Verification items for the finished model (mm, model axes). Give positions to 0.01 mm unless a question says otherwise; leave off trailing zeros. Loops run counter-clockwise (first coordinate to the right, second up) from the corner with the lowest first, then second, coordinate; pieces in that order, holes last. Notation, with made-up numbers: M -36,-10 L -7,-10 A29 ccw -7,17 Z; hole C 49,10.25 d2. An arc over 180 degrees is marked long. Use CSV: the item, a comma, the result in double quotes.
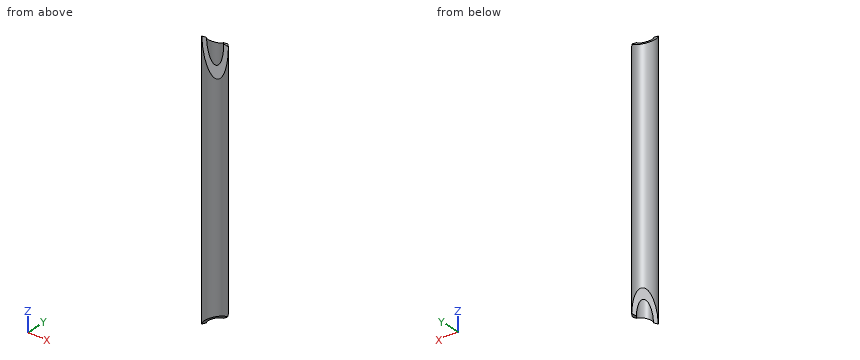
Autodesk Inventor part; units mm, degrees
ref_plane "Start Plane" through (0, 0, -3.37) normal (0, 0, 1) x (1, 0, 0)
ref_plane "End Plane" through (0, 0, 266.7183) normal (0, 0, 1) x (1, 0, 0)
ref_plane "Work Plane4" through (-6.8383, -8.1881, -6.8069) normal (0.3448, 0.4129, -0.843) x (0.2427, -0.9068, -0.3448)
ref_plane "Start Plane" through (0, 0, -3.37) normal (0, 0, 1) x (1, 0, 0)
ref_plane "End Plane" through (0, 0, 266.7183) normal (0, 0, 1) x (1, 0, 0)
sketch "Sketch" plane through (0, 0, 0) normal (0, 0, 1) x (1, 0, 0)
  circle A0 centre (0, 0) radius 6.9342
  circle A1 centre (0, 0) radius 10.668
  dimension "d0" = 21.336
  dimension "d1" = 3.7338
extrude "Body" add sketch "Sketch" along normal up to surface (270.0883 mm away) from surface at -3.37
sketch "Sketch3" plane through (0, 0, 0) normal (0, 0, 1) x (1, 0, 0)
  line L0 (0, 0) -> (10, 0)
ref_plane "Work Plane3" through (0, 0, 0) normal (0, -1, 0) x (1, 0, 0)
sketch "Sketch4" plane through (0, 0, 0) normal (0, -1, 0) x (1, 0, 0)
  line L0 (-2, -3.37) -> (12, -3.37)
  line L1 (-2, 266.7183) -> (12, 266.7183)
  dimension "d7" = 270.0883
ref_plane "Work Plane4" through (-6.8383, -8.1881, -6.8069) normal (0.3448, 0.4129, -0.843) x (0.2427, -0.9068, -0.3448)
split "Split1" plane through (-6.8383, -8.1881, -6.8069) removes the side toward (0.3448, 0.4129, -0.843)
ref_plane "Work Plane5" through (4.7044, -9.5747, -24.7602) normal (-0.405, 0.8243, -0.3957) x (0.7286, 0.5524, 0.405)
split "Split2" plane through (4.7044, -9.5747, -24.7602) removes the side toward (-0.405, 0.8243, -0.3957)
ref_plane "Work Plane6" through (-8.4798, 6.473, -10.5353) normal (0.5585, -0.4264, -0.7115) x (-0.0814, 0.8255, -0.5585)
split "Split3" plane through (-8.4798, 6.473, -10.5353) removes the side toward (0.5585, -0.4264, -0.7115)
ref_plane "Work Plane7" through (3.7346, -9.993, 272.7308) normal (-0.242, 0.6474, 0.7227) x (0.966, 0.0909, 0.242)
split "Split4" plane through (3.7346, -9.993, 272.7308) removes the side toward (-0.242, 0.6474, 0.7227)
ref_plane "Work Plane8" through (-8.4798, 6.473, 292.9957) normal (0.7502, -0.5727, 0.3305) x (0.577, 0.3229, -0.7502)
split "Split5" plane through (-8.4798, 6.473, 292.9957) removes the side toward (0.7502, -0.5727, 0.3305)
ref_plane "Work Plane9" through (-10.6242, -0.9653, 270.4444) normal (0.5935, 0.0539, 0.8031) x (0.8047, -0.0177, -0.5935)
split "Split6" plane through (-10.6242, -0.9653, 270.4444) removes the side toward (0.5935, 0.0539, 0.8031)
equation "\"d0\" = G_H"
equation "\"d1\" = G_T"
equation "\"d2\" = G_L"
equation "\"G_H\" = 21.336"
equation "\"G_T\" = 3.7338"
equation "\"G_L\" = 270.08826"
equation "\"G_OFFSET_START\" = 3.36995"
equation "\"G_OFFSET_END\" = 4.18997"
equation "\"d4\" = -G_OFFSET_START"
equation "\"d5\" = G_OFFSET_END + B_L"
equation "\"B_L\" = 262.52833"
properties part number "ANSI - 1/2 x 0.147 - 10.633" material "Steel, Mild"
(1) Scan lines: L1, parallel to X at y = 0, z = 73; L2, parallel to Y at x = -2, z = 64.5. Record each from-to range of solid material in increasing order. Write a range as from..to.
Calculated:
L1,"x = -10.67..-6.93, 6.93..10.67"
L2,"y = -10.48..-6.64, 6.64..10.48"
(2) Section check A-A on x = -2.5. Record the cut outline in (y, z).
Calculated:
outline,"M -10.37,4.25 L -6.47,1.91 L -6.47,257 L -10.37,250.23 Z; M 6.47,16.03 L 10.37,24.16 L 10.37,252.4 L 6.47,255.9 Z"
(3) Section check B-B on y = 0. Record the cut outline in (x, z), plus the area to 3 significant figures.
Calculated:
outline,"M -10.67,10.92 L -6.93,7.1 L -6.93,260.21 L -10.67,258.96 Z; M 6.93,5.44 L 10.67,8.37 L 10.67,238.32 L 6.93,246.79 Z"
area,"1,820 mm²"
(4) Depth check by flat-ended pin: pin 1 Ø3 at (x, z) = (-1.5, 31) entering from -Y; pin 2 Ø12 at (y, z) = (6.5, 175.5) entering from +X; pin 3 Ø3 at (y, z) = (7.5, 237.5) entering from +X; pin 4 Ø3 at (x, z) = (6.5, 217.5) entering from +Y. Enter the tip coordinate at first touch or a pass-through.
Calculated:
pin 1,"stops at y = -10.67"
pin 2,"stops at x = 10.66"
pin 3,"stops at x = 8.82"
pin 4,"stops at y = 9.42"
(5) Section check C-C on z = 158.5. Record the cut outline in (x, y), plus the area to 3 significant figures.
Calculated:
outline,"C 0,0 d21.34; hole C 0,0 d13.87"
area,"206 mm²"
